from build123d import *

# Parameters (mm, degrees)
SKETCH1_R           = 22.335
BOSS_EXTRUDE1_DEPTH = 112
CUT_EXTRUDE1_START  = -9
SKETCH2_R           = 22.335
SKETCH2_R_2         = 20
CUT_EXTRUDE1_DEPTH  = 9
SKETCH3_R           = 22.335
SKETCH3_R_2         = 20
CUT_EXTRUDE2_DEPTH  = 99
CUT_EXTRUDE3_START  = 4.5
SKETCH4_R           = 22.335
SKETCH4_R_2         = 19.5
CUT_EXTRUDE3_DEPTH  = 4.5
SKETCH5_R           = 16
CUT_EXTRUDE4_DEPTH  = 10
CHAMFER1_SIZE       = 0.5
SKETCH6_R           = 7.5
CUT_EXTRUDE5_DEPTH  = 107.77876404
CUT_EXTRUDE6_START  = -92.45
SKETCH6_2_R         = 16
SKETCH6_2_R_2       = 7.5
CUT_EXTRUDE6_DEPTH  = 15.32876404
CHAMFER2_SIZE       = 2
CUT_EXTRUDE8_START  = -12
SKETCH8_R           = 16
CUT_EXTRUDE8_DEPTH  = 12
CHAMFER3_SIZE       = 1
CUT_EXTRUDE9_START  = -85
CUT_EXTRUDE9_DEPTH  = 85
CUT_EXTRUDE10_REACH = 118.982
CUT_EXTRUDE11_DEPTH = 117.368829375
LPATTERN1_COUNT     = 15
LPATTERN1_PITCH     = 5


# Read off the part's stored shape, not the designer's step: Cut-Extrude9
with BuildPart() as part:
    # Sketch1 → Boss-Extrude1 (new body)
    with BuildSketch(Plane.XY):
        Circle(SKETCH1_R)
    extrude(amount=BOSS_EXTRUDE1_DEPTH)

    # Sketch2 → Cut-Extrude1 (cut)
    with BuildSketch(Plane.XY.offset(112).offset(CUT_EXTRUDE1_START)):
        Circle(SKETCH2_R)
        Circle(SKETCH2_R_2, mode=Mode.SUBTRACT)
    extrude(amount=CUT_EXTRUDE1_DEPTH, mode=Mode.SUBTRACT)

    # Sketch3 → Cut-Extrude2 (cut)
    with BuildSketch(Plane(origin=(0, 0, 0), x_dir=(-1, 0, 0), z_dir=(0, 0, -1))):
        Circle(SKETCH3_R)
        with Locations(Location((0, 0, 0), (0, 0, 180))):
            Circle(SKETCH3_R_2, mode=Mode.SUBTRACT)
    extrude(amount=-CUT_EXTRUDE2_DEPTH, mode=Mode.SUBTRACT)

    # Sketch4 → Cut-Extrude3 (cut)
    with BuildSketch(Plane(origin=(0, 0, 99), x_dir=(-1, 0, 0), z_dir=(0, 0, -1)).offset(CUT_EXTRUDE3_START)):
        Circle(SKETCH4_R)
        Circle(SKETCH4_R_2, mode=Mode.SUBTRACT)
    extrude(amount=-CUT_EXTRUDE3_DEPTH, mode=Mode.SUBTRACT)

    # Sketch5 → Cut-Extrude4 (cut)
    with BuildSketch(Plane.XY.offset(112)):
        Circle(SKETCH5_R)
    extrude(amount=-CUT_EXTRUDE4_DEPTH, mode=Mode.SUBTRACT)

    # Chamfer1
    chamfer1_edges = [part.edges().sort_by_distance(p)[0] for p in [
        (-16, 0, 112),
        (-20, 0, 112),
    ]]
    chamfer(chamfer1_edges, length=CHAMFER1_SIZE)

    # Sketch6 → Cut-Extrude5 (cut, through all)
    with BuildSketch(Plane.XY.offset(102)):
        Circle(SKETCH6_R)
    extrude(amount=-CUT_EXTRUDE5_DEPTH, mode=Mode.SUBTRACT)

    # Sketch6<2> → Cut-Extrude6 (cut, through all)
    with BuildSketch(Plane.XY.offset(102).offset(CUT_EXTRUDE6_START)):
        Circle(SKETCH6_2_R)
        Circle(SKETCH6_2_R_2, mode=Mode.SUBTRACT)
    extrude(amount=-CUT_EXTRUDE6_DEPTH, mode=Mode.SUBTRACT)

    # Chamfer2
    chamfer2_edges = [part.edges().sort_by_distance(p)[0] for p in [
        (-20, 0, 0),
    ]]
    chamfer(chamfer2_edges, length=CHAMFER2_SIZE)

    # Sketch8 → Cut-Extrude8 (cut)
    with BuildSketch(Plane(origin=(0, 0, 0), x_dir=(-1, 0, 0), z_dir=(0, 0, -1)).offset(CUT_EXTRUDE8_START)):
        with Locations(Location((0, 0, 0), (0, 0, 180))):
            Circle(SKETCH8_R)
    extrude(amount=CUT_EXTRUDE8_DEPTH, mode=Mode.SUBTRACT)

    # Chamfer3
    chamfer3_edges = [part.edges().sort_by_distance(p)[0] for p in [
        (-16, 0, 0),
    ]]
    chamfer(chamfer3_edges, length=CHAMFER3_SIZE)

    # Cut-Extrude9 outline → Cut-Extrude9 (cut)
    with BuildSketch(Plane(origin=(0, 0, 0), x_dir=(-1, 0, 0), z_dir=(0, 0, -1)).offset(CUT_EXTRUDE9_START)):
        with BuildLine():
            Line((3, 17.903719933), (3, 19.773719933))
            ThreePointArc((3, 19.773719933), (0, 20), (-3, 19.773719933))
            Line((-3, 19.773719933), (-3, 17.903719933))
            Line((-3, 17.903719933), (-1.859250535, 17.903719933))
            ThreePointArc((-1.859250535, 17.903719933), (0, 18), (1.859250535, 17.903719933))
            Line((1.859250535, 17.903719933), (3, 17.903719933))
        make_face()
    extrude(amount=CUT_EXTRUDE9_DEPTH, mode=Mode.SUBTRACT)

    # Cut-Extrude10: up to this face of the body (flat: up to its plane)
    cut_extrude10_end = Plane(part.part.faces().sort_by_distance((3, 18.835290902, 43.036448518))[0])
    # Sketch11 → Cut-Extrude10 (cut, up to the picked face)
    with BuildSketch(Plane(origin=(-3, 0, 0), x_dir=(0, 0, -1), z_dir=(1, 0, 0)), mode=Mode.PRIVATE) as cut_extrude10_sk1:
        Polygon((-93, 20), (-85, 20), (-85, 17.903719933), align=None)
    cut_extrude10_tool1 = split(extrude(cut_extrude10_sk1.sketch, amount=CUT_EXTRUDE10_REACH, mode=Mode.PRIVATE), bisect_by=cut_extrude10_end, keep=Keep.BOTH, mode=Mode.PRIVATE)
    add(cut_extrude10_tool1.solids().sort_by(Axis((-3, 19.30124, 87.666667), (1, 0, 0)))[0], mode=Mode.SUBTRACT)

    # Sketch13 → Cut-Extrude11 (cut, symmetric)
    with BuildSketch(Plane(origin=(0, 0, 0), x_dir=(1, 0, 0), z_dir=(0, 1, 0))):
        Polygon((17.3, -83), (17.3, -84), (22.7, -86), (22.7, -81), align=None)
    cut_extrude11 = extrude(amount=CUT_EXTRUDE11_DEPTH, both=True, mode=Mode.SUBTRACT)

    # LPattern1: Cut-Extrude11 ×15
    with Locations(*[(0, 0, -i * LPATTERN1_PITCH) for i in range(1, LPATTERN1_COUNT)]):
        add(cut_extrude11, mode=Mode.SUBTRACT)


solid = part.part
Read the model definition and answer for the solid it produces. Units are mm, in the model's axes. A direction names the side the tool comes from. Round coordinates to 2 decimals unless told otherwise and drop trailing zeros.
1) For faces 5 (the face through (0.779, -18.303, 0.319)), 6 (the face through (-17, -11, 103)), 7 (the face through (18.369, 0.14, 17.604)), determine the directions among +Z, -Z, +X, -X, +Y, -Y from which every point of the face is accessible in a straight line to the end or side of a thin tool.
2) The mould has two halves that part along Y. Classify faces 1 (the face through (6.89, -3.33, 102)), 2 (the face through (0, -20, 99)), 3 (the face through (0, 18, 43)), 4 (the face through (-3.47, -15.62, 106.82)): released by +Y, released by -Y, zero draft, split by the parting line, or undercut.
3) Flat-ended cylindrical pins translate along their axes: pin 1 (1.5 mm diameter, centred on y = 5.5, z = 20, fed in from -X); pin 2 (1.3 mm diameter, centred on x = 2, z = 24.5, fed in from +Y); pin 3 (8 mm diameter, centred on y = 14, z = 49.5, fed in from -X); pin 4 (12 mm diameter, centred on x = -16, y = -12.5, fed in from +Z). Find the tip coordinate at first contact, or state that the pin passes through.
4) Straight lines are drawn through the part: L1, parallel to Y at x = 0, z = 58; L2, parallel to Z at x = -11.5, y = 4.5; L3, parallel to Z at x = -11, y = -15.5. For each, find the intervals that lie inside material, in ascending order.
Resolved:
1. face 5: -Z
1. face 6: +Z
1. face 7: +X, +Y, -Y
2. face 1: undercut
2. face 2: zero draft
2. face 3: released by +Y
2. face 4: undercut
3. pin 1: stops at x = -19.43
3. pin 2: stops at y = 17.95
3. pin 3: stops at x = -17.32
3. pin 4: stops at z = 112
4. L1: y = -20 to -7.5, 7.5 to 18
4. L2: z = 12 to 102
4. L3: z = 1.01 to 112
